Verification items for the finished model (mm, model axes). Round coordinates to 2 decimals unless told otherwise and drop trailing zeros. Write each loop counter-clockwise with the first axis right and the second up, starting at its lowest first coordinate (ties: lowest second). Pieces come first, ordered by that corner, then holes. Notation, with made-up numbers: (-13, 33.5) - (15, 33.5) arc R24 ccw to (15, 72.5) - close; hole circle Ø10 at (29.5, -22). An arc over 180 degrees is marked (long way). Answer as a JSON object with one key per item and string values. Group by question number.
1) Section check A-A (y = 284.5). Enter the section's corners in (x, z), then the cut area to 3 significant figures.
2) Thickness scan on line 1 (Z direction, x = -13.25, y = 288.5); line 2 (Y direction, x = -1, z = 1719.5). Record the ranges inside material, lowest first.
3) Section check B-B (x = -11). Enter the section's corners in (y, z).
```python
from build123d import *

# Parameters (mm, degrees)
F0_W     = 650
F0_H     = 2430
F1_DEPTH = 18
F2_W     = 390
F2_H     = 445
F3_DEPTH = 18.001


with BuildPart() as f1:
    # F0 (on Right) → F1 (new body)
    with BuildSketch(Plane.YZ):
        with Locations((325, 1215)):
            Rectangle(F0_W, F0_H)
    extrude(amount=-F1_DEPTH)

    # F2 (on face) → F3 (cut, through all)
    with BuildSketch(Plane.YZ):
        with Locations((325, 1852)):
            Rectangle(F2_W, F2_H)
    extrude(amount=-F3_DEPTH, mode=Mode.SUBTRACT)


solid = f1.part
```
Returned:
{
 "1": {"outline": "(-18, 0) - (0, 0) - (0, 1629.5) - (-18, 1629.5) - close; (-18, 2074.5) - (0, 2074.5) - (0, 2430) - (-18, 2430) - close", "area": "35,700 mm2"},
 "2": {"line 1": "0 to 1629.5, 2074.5 to 2430", "line 2": "0 to 130, 520 to 650"},
 "3": {"outline": "(0, 0) - (650, 0) - (650, 2430) - (0, 2430) - close; hole (130, 1629.5) - (520, 1629.5) - (520, 2074.5) - (130, 2074.5) - close"}
}
